Autodesk Inventor part; units mm, degrees
ref_plane "YZ Plane" through (0, 0, 0) normal (1, 0, 0) x (0, 1, 0)
ref_plane "XZ Plane" through (0, 0, 0) normal (0, 1, 0) x (-1, 0, 0)
ref_plane "XY Plane" through (0, 0, 0) normal (0, 0, 1) x (1, 0, 0)
sketch "Sketch1" plane through (0, 0, 0) normal (0, 1, 0) x (-1, 0, 0)
  circle A0 centre (0, 0) radius 166.37
  dimension "d0" = 332.74
extrude "Extrusion1" add sketch "Sketch1" along normal blind 152.4
sketch "Sketch2" plane through (0, 152.4, 0) normal (0, 1, 0) x (1, 0, 0)
  circle A0 centre (0, 0) radius 163.83
  dimension "d3" = 327.66
extrude "Extrusion2" cut sketch "Sketch2" against normal blind 147.32
fillet "Fillet1" radius 12.7 1 edges at (166.37, 0, 0)
properties part number "cover" material "Acetal Resin, White"
Model file for the job. Use its own axes, mm. Round coordinates to 2 decimals unless told otherwise and drop trailing zeros. Loops run counter-clockwise (first coordinate to the right, second up) from the corner with the lowest first, then second, coordinate; pieces in that order, holes last.
1. Mould opens along Z. For faces 1 (the cylindrical face through (-35.515, 79.771, 159.934)), 2 (the cylindrical face through (21.658, 81.572, -164.954)), 3 (the flat face through (-122, 152.4, -110)), 4 (the flat face through (-2, 5.08, -2)) say: +Z half, -Z half, draft (parallel to the pull), parting line (faces both ways), or undercut.
Check values:
face 1: undercut
face 2: parting line
face 3: draft
face 4: undercut
2. Wall check: probe 1 along Z at (x, y) = (0, 63); probe 2 along Y at (x, z) = (-55.5, 104); probe 3 along Z at (x, y) = (65.5, 62.5). Give the ranges that are in metal, low to high.
Check values:
probe 1: z = -166.37 to -163.83, 163.83 to 166.37
probe 2: y = 0 to 5.08
probe 3: z = -152.93 to -150.17, 150.17 to 152.93
3. Drop flat-ended pins along their axis: P1, Ø1, axis at x = 58.5, y = 73.5, coming from the +Z side; P2, Ø3, axis at x = -103.5, y = 62.5, coming from the +Z side; P3, Ø10, axis at y = 63.5, z = 91.5, coming from the +X side. Give the stop position or say it passes through.
Check values:
P1: stops at z = 155.93
P2: stops at z = 131.43
P3: stops at x = 142.12
4. Band-saw the part on B-B, the plane y = 44. List the corners of the cut face in (x, z).
Check values:
outline: circle Ø332.74 at (0, 0); hole circle Ø327.66 at (0, 0)
